```python
from build123d import *

# Parameters (mm, degrees)
SKETCH001_W  = 120
SKETCH001_H  = 76
SKETCH001_R  = 1.5
PAD_DEPTH    = 10
SKETCH_W     = 70
SKETCH_H     = 76
PAD001_DEPTH = 10


with BuildPart() as part:
    # Sketch001 → Pad (new body)
    with BuildSketch(Plane.YZ):
        with Locations((-60, 0)):
            Rectangle(SKETCH001_W, SKETCH001_H)
        with Locations((-82.756082, 32)):
            Circle(SKETCH001_R, mode=Mode.SUBTRACT)
        with Locations((-114.756082, 0)):
            Circle(SKETCH001_R, mode=Mode.SUBTRACT)
        with Locations((-50.756082, 0)):
            Circle(SKETCH001_R, mode=Mode.SUBTRACT)
        with Locations((-82.756082, -32)):
            Circle(SKETCH001_R, mode=Mode.SUBTRACT)
    extrude(amount=PAD_DEPTH)

    # Sketch → Pad001 (join)
    with BuildSketch(Plane.XZ):
        with Locations((35, 0)):
            Rectangle(SKETCH_W, SKETCH_H)
    extrude(amount=PAD001_DEPTH)


solid = part.part
```
Can you work these out from the model? Positions are in its coordinate system, mm. A direction names the side the tool comes from. Give positions to 0.01 mm unless a question says otherwise; leave off trailing zeros. Loops run counter-clockwise (first coordinate to the right, second up) from the corner with the lowest first, then second, coordinate; pieces in that order, holes last. Notation, with made-up numbers: M 16.25,59.25 L 64.25,59.25 A18 ccw 64.25,94.25 Z; hole C -26.75,-14.75 d5. An arc over 180 degrees is marked long. One line per item, written item: value.
(1) Suppose I cut it at D-D on x = 32.5. List the corners of the cut face in (y, z) for me, plus the area to 3 significant figures.
Returned:
outline: M -10,-38 L 0,-38 L 0,38 L -10,38 Z
area: 760 mm^2
(2) We'd pull the mould along Z, two halves only. Please class faces 3 (the face through (9, -43, -38)), 4 (the face through (4.93, -84.255, -31.934)), 5 (the face through (70, -5, -1)): released by +Z, released by -Z, zero draft, split by the parting line, or undercut.
Returned:
face 3: released by -Z
face 4: undercut
face 5: zero draft
(3) I need wall thicknesses on line 1 (X direction, y = -28.5, z = -30.5); line 2 (Y direction, x = 62, z = -15.5). Which ranges of each line are inside material? Lowest first, please.
Returned:
line 1: 0 to 10
line 2: -10 to 0
(4) Suppose I cut it at A-A on z = 0. List the corners of the cut face in (x, y) for me.
Returned:
outline: M 0,-120 L 10,-120 L 10,-116.26 L 0,-116.26 Z; M 0,-113.26 L 10,-113.26 L 10,-52.26 L 0,-52.26 Z; M 0,-49.26 L 10,-49.26 L 10,-10 L 70,-10 L 70,0 L 0,0 Z
(5) Which directions (+Z, -Z, +X, -X, +Y, -Y) give clear straight access to the entire face, cutting with the end or side of a thin tool? Please do faces 1 (the face through (10, -66, 1)), 2 (the face through (9, -43, 38)).
Returned:
face 1: +Z, -Z, +X, -Y
face 2: +Z, +X, -X, +Y, -Y
(6) Suppose I cut it at B-B on z = -32. List the corners of the cut face in (x, y) for me.
Returned:
outline: M 0,-120 L 10,-120 L 10,-84.26 L 0,-84.26 Z; M 0,-81.26 L 10,-81.26 L 10,-10 L 70,-10 L 70,0 L 0,0 Z
(7) Will these pins go through, and if not, where does the flat tip stop? pin 1 (1.5 mm diameter, centred on x = 11, y = -39, fed in from -Z); pin 2 (4 mm diameter, centred on y = -68, z = -26.5, fed in from +X); pin 3 (3 mm diameter, centred on x = 57, z = 4, fed in from -Y).
Returned:
pin 1: through
pin 2: x = 10
pin 3: y = -10
(8) Suppose I cut it at C-C on y = -46. List the corners of the cut face in (x, z) for me, plus the area to 3 significant figures.
Returned:
outline: M 0,-38 L 10,-38 L 10,38 L 0,38 Z
area: 760 mm^2
